from build123d import *

# Parameters (mm, degrees)
SKETCH1_W           = 7.6
SKETCH1_H           = 7.4
BOSS_EXTRUDE1_DEPTH = 6
BOSS_EXTRUDE2_DEPTH = 7.6
SKETCH3_W           = 2
SKETCH3_H           = 2
CUT_EXTRUDE1_DEPTH  = 6


with BuildPart() as part:
    # Sketch1 → Boss-Extrude1 (new body)
    with BuildSketch(Plane.XY):
        Rectangle(SKETCH1_W, SKETCH1_H)
    extrude(amount=BOSS_EXTRUDE1_DEPTH)

    # Sketch2 → Boss-Extrude2 (add)
    with BuildSketch(Plane(origin=(3.8, 0, 0), x_dir=(0, 0, -1), z_dir=(1, 0, 0))):
        Polygon((-6, 3.7), (-6, -3.7), (-7, -3.7), (-7, -3.2), (-9.8, -2.5), (-9.8, 1.7), align=None)
    extrude(amount=-BOSS_EXTRUDE2_DEPTH)

    # Sketch3 → Cut-Extrude1 (cut)
    with BuildSketch(Plane(origin=(0, 3.7, 0), x_dir=(1, 0, 0), z_dir=(0, 1, 0))):
        with Locations((-1.8, -2.2)):
            Rectangle(SKETCH3_W, SKETCH3_H)
        with Locations((1.8, -2.2)):
            Rectangle(SKETCH3_W, SKETCH3_H)
    extrude(amount=-CUT_EXTRUDE1_DEPTH, mode=Mode.SUBTRACT)


solid = part.part
Design review of the part built by this model. Coordinates are the model's own, in mm. A direction names the side the tool comes from. Round coordinates to 2 decimals unless told otherwise and drop trailing zeros. Loops run counter-clockwise (first coordinate to the right, second up) from the corner with the lowest first, then second, coordinate; pieces in that order, holes last. Notation, with made-up numbers: (53.5, 7.25) -> (106.5, 7.25) arc R33 cw to (106.5, 37.25) -> close; hole circle Ø6 at (79.25, 41). An arc over 180 degrees is marked (long way). Use one line per item in the form item = value. Start each with the question number.
Q1. Wall thickness on line 1 along X through (y, z) = (2.5, 2); line 2 along Z through (x, y) = (-1.5, -2); line 3 along Z through (x, y) = (-2.5, 3.25) (3 decimals): over which ranges is each line inside the solid? List them lowest first. Write a range as [from, to].
Q2. Machinability: for faces 1 (the face through (0, -3.7, 3)), 2 (the face through (2, 1, 3.2)), which of the approach directions +Z, -Z, +X, -X, +Y, -Y give a long, thin tool a straight path to every point of the face, cutting with its end or side? Answer none if there is none.
Q3. For pin 1 Ø0.6 at (x, z) = (-2, 2) entering from +Y, flat-tipped, find the tip position at first contact; note if it passes through.
Q4. We need section C-C on x = 1.5. Give the boundary of the cut face in (y, z), then the cut area to 3 significant figures.
Q5. We need section B-B on z = 1.5. Give the boundary of the cut face in (x, y), then the cut area to 3 significant figures.
Q6. We need section D-D on y = 0.75. Give the boundary of the cut face in (x, z), then the cut area to 3 significant figures.
Q7. Draft analysis for pull direction X (two halves, no side actions). For faces 3 (the face through (0.053, -2.855, 8.38)), 4 (the face through (-0.8, 1, 2)), 5 (the face through (3.8, 0, 5)), state which applies: +X half, -X half, draft (parallel to the pull), parting line (faces both ways), or undercut.
Q8. We need section A-A on y = 2. Give the boundary of the cut face in (x, z), then the cut area to 3 significant figures.
Calculated:
q1.line_1 = [-3.8, -2.8], [-0.8, 0.8], [2.8, 3.8]
q1.line_2 = [0, 1.2], [3.2, 9.8]
q1.line_3 = [0, 1.2], [3.2, 6.855]
q2.face_1 = +Z, -Z, +X, -X, -Y
q2.face_2 = +Y
q3.pin_1 = -2.3
q4.outline = (-3.7, 0) -> (3.7, 0) -> (3.7, 1.2) -> (-2.3, 1.2) -> (-2.3, 3.2) -> (3.7, 3.2) -> (3.7, 6) -> (1.7, 9.8) -> (-2.5, 9.8) -> (-3.2, 7) -> (-3.7, 7) -> close
q4.area = 54.3 mm²
q5.outline = (-3.8, -3.7) -> (3.8, -3.7) -> (3.8, 3.7) -> (2.8, 3.7) -> (2.8, -2.3) -> (0.8, -2.3) -> (0.8, 3.7) -> (-0.8, 3.7) -> (-0.8, -2.3) -> (-2.8, -2.3) -> (-2.8, 3.7) -> (-3.8, 3.7) -> close
q5.area = 32.2 mm²
q6.outline = (-3.8, 0) -> (3.8, 0) -> (3.8, 9.8) -> (-3.8, 9.8) -> close; hole (-2.8, 1.2) -> (-0.8, 1.2) -> (-0.8, 3.2) -> (-2.8, 3.2) -> close; hole (0.8, 1.2) -> (2.8, 1.2) -> (2.8, 3.2) -> (0.8, 3.2) -> close
q6.area = 66.5 mm²
q7.face_3 = draft
q7.face_4 = undercut
q7.face_5 = +X half
q8.outline = (-3.8, 0) -> (3.8, 0) -> (3.8, 9.23) -> (-3.8, 9.23) -> close; hole (-2.8, 1.2) -> (-0.8, 1.2) -> (-0.8, 3.2) -> (-2.8, 3.2) -> close; hole (0.8, 1.2) -> (2.8, 1.2) -> (2.8, 3.2) -> (0.8, 3.2) -> close
q8.area = 62.1 mm²
